Print and shaded views of the part. All mm, measured from the part's lowest x, y and z. A direction names the side the tool comes from. Round coordinates to 2 decimals unless told otherwise and drop trailing zeros. Write each loop counter-clockwise with the first axis right and the second up, starting at its lowest first coordinate (ties: lowest second). Pieces come first, ordered by that corner, then holes.
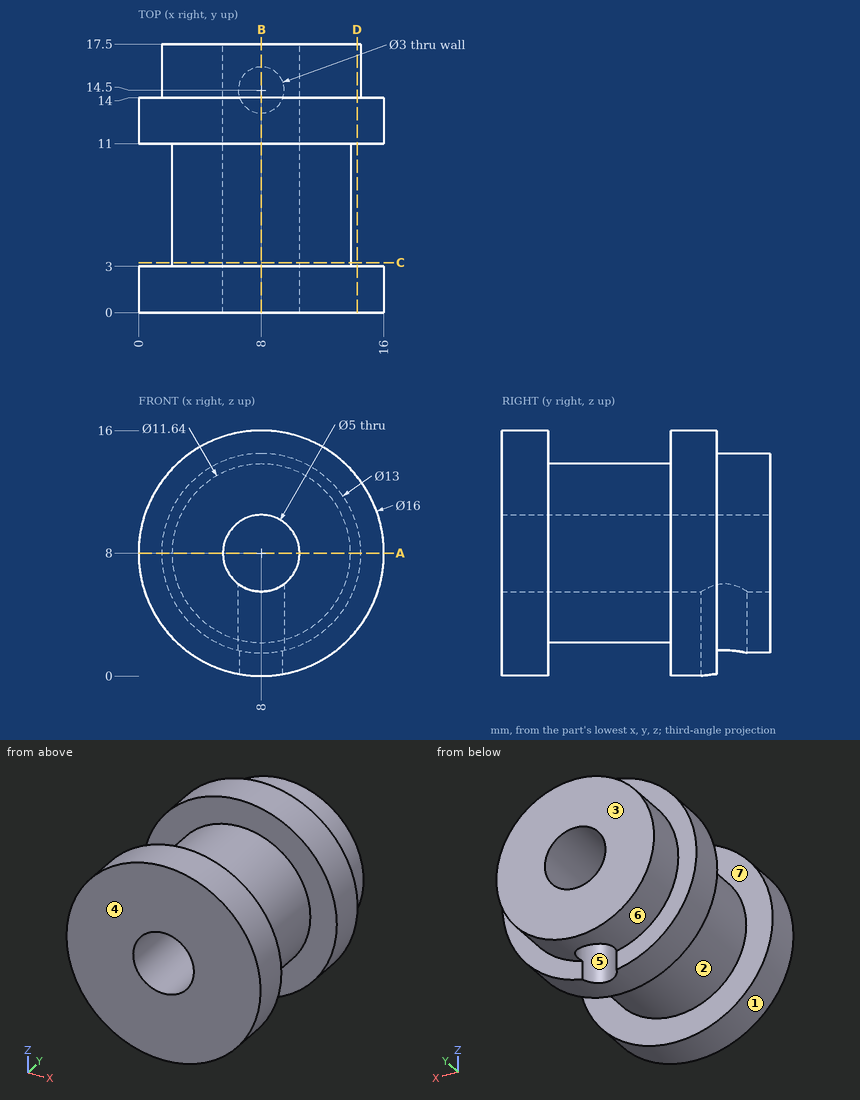
1) Slice it at C-C (y = 3.25). Write the cut outline in (x, z).
Results:
outline: circle Ø11.64 at (8, 8); hole circle Ø5 at (8, 8)
2) Mould opens along Y. For the marked faces 1, 2, 3 and 4 say: released by +Y, released by -Y, zero draft, split by the parting line, or undercut.
Results:
face 1: zero draft
face 2: undercut
face 3: released by +Y
face 4: released by -Y
3) Wall check: L1, parallel to X at y = 13, z = 8; L2, parallel to X at y = 10, z = 8; L3, parallel to Y at x = 12, z = 3.5. Give the ranges that are in metal, low to high.
Results:
L1: x = 0 to 5.5, 10.5 to 16
L2: x = 2.18 to 5.5, 10.5 to 13.82
L3: y = 0 to 3, 11 to 17.5
4) Slice it at B-B (x = 8). Write the cut outline in (y, z), plus the area to 3 significant figures.
Results:
outline: (0, 0) - (3, 0) - (3, 2.18) - (11, 2.18) - (11, 0) - (13, 0) - (13, 5.5) - (0, 5.5) - close; (0, 10.5) - (17.5, 10.5) - (17.5, 14.5) - (14, 14.5) - (14, 16) - (11, 16) - (11, 13.82) - (3, 13.82) - (3, 16) - (0, 16) - close; (16, 1.5) - (17.5, 1.5) - (17.5, 5.5) - (16, 5.5) - close
area: 134 mm2
5) Slice it at D-D (x = 14.25). Write the cut outline in (y, z).
Results:
outline: (0, 3.01) - (3, 3.01) - (3, 12.99) - (0, 12.99) - close; (11, 3.01) - (14, 3.01) - (14, 6.21) - (17.5, 6.21) - (17.5, 9.79) - (14, 9.79) - (14, 12.99) - (11, 12.99) - close
6) Slice it at A-A (z = 8). Write the cut outline in (x, y).
Results:
outline: (0, 0) - (5.5, 0) - (5.5, 17.5) - (1.5, 17.5) - (1.5, 14) - (0, 14) - (0, 11) - (2.18, 11) - (2.18, 3) - (0, 3) - close; (10.5, 0) - (16, 0) - (16, 3) - (13.82, 3) - (13.82, 11) - (16, 11) - (16, 14) - (14.5, 14) - (14.5, 17.5) - (10.5, 17.5) - close
7) Pin check, flat tips, straight feed: pin 1 Ø5 at (x, y) = (11.5, 13) entering from -Z; pin 2 Ø1 at (x, y) = (3.5, 12) entering from -Z; pin 3 Ø1.5 at (y, z) = (7.5, 5) entering from +X; pin 4 Ø4 at (x, z) = (8, 8) entering from +Y. Stop position of each tip, or through.
Results:
pin 1: stops at z = 0.06
pin 2: stops at z = 1.07
pin 3: stops at x = 13.37
pin 4: passes through
8) Which spindle directions (+Z, -Z, +X, -X, +Y, -Y) get a long thin tool onto all of the face, cutting with end or side? Do the marked faces 5, 6 and 7. Say none if no direction does.
Results:
face 5: -Z
face 6: +Y
face 7: none
